Drawing for the job (mm, zero at the part's lowest x, y, z). A direction names the side the tool comes from. Coordinates: 2 decimals unless noted, no trailing zeros. Write each loop counter-clockwise with the first axis right and the second up, starting at its lowest first coordinate (ties: lowest second). Pieces come first, ordered by that corner, then holes. Notation, with made-up numbers: M 41,84 L 98,84 A24 ccw 98,104 Z; hole C 11.25,-19 d3. An arc over 180 degrees is marked long. Put each result on its own line as item: value. Start each with the question number.
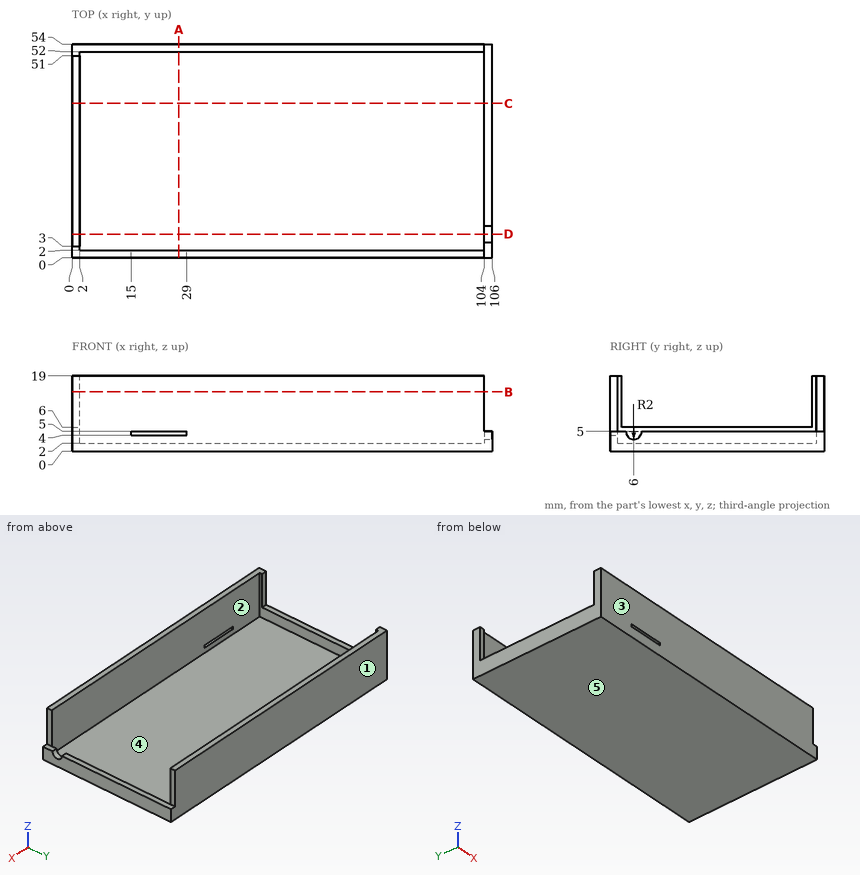
(1) Slice it at D-D, the plane y = 6. Write the cut outline in (x, z).
(2) Slice it at A-A, the plane x = 27. Write the cut outline in (y, z), then the cut area to 3 significant figures.
(3) Two-plate mould, pull along Y, no slides. Class the marked faces 1, 2 and 3: +Y half, -Y half, draft (parallel to the pull), parting line (faces both ways), or undercut.
(4) Which spindle directions (+Z, -Z, +X, -X, +Y, -Y) get a long thin tool onto all of the face, cutting with end or side? Do the marked faces 4 and 5. Say none if no direction does.
(5) Drop flat-ended pins along their axis: pin 1 (1.6 mm diameter, centred on x = 1.5, z = 15.5, fed in from -Y); pin 2 (1 mm diameter, centred on x = 66.5, y = 33.5, fed in from +Z); pin 3 (1.6 mm diameter, centred on x = 105.5, y = 41, fed in from +Z); pin 4 (2 mm diameter, centred on y = 53, z = 11.5, fed in from +X). Give the stop position or say it passes through.
(6) Slice it at C-C, the plane y = 39. Write the cut outline in (x, z), then the cut area to 3 significant figures.
(7) Drill centre lines: line 1 (Y direction, x = 88, z = 4); line 2 (Z direction, x = 99, y = 36). Where is each one in solid material? Low to high. Write a range as [from, to].
(8) Slice it at B-B, the plane z = 15. Write the cut outline in (x, y), then the cut area to 3 significant figures.
Result set:
1. outline: M 0,0 L 106,0 L 106,3 L 104,3 L 104,2 L 2,2 L 2,6 L 0,6 Z
2. outline: M 0,0 L 54,0 L 54,19 L 52,19 L 52,2 L 2,2 L 2,4 L 0,4 Z; M 0,5 L 2,5 L 2,19 L 0,19 Z
2. area: 174 mm^2
3. face 1: +Y half
3. face 2: undercut
3. face 3: -Y half
4. face 4: +Z
4. face 5: -Z, +X, -X, +Y, -Y
5. pin 1: stops at y = 0
5. pin 2: stops at z = 2
5. pin 3: stops at z = 5
5. pin 4: stops at x = 104
6. outline: M 0,0 L 106,0 L 106,5 L 104,5 L 104,2 L 2,2 L 2,6 L 0,6 Z
6. area: 226 mm^2
7. line 1: y = [0, 2], [52, 54]
7. line 2: z = [0, 2]
8. outline: M 0,0 L 104,0 L 104,2 L 2,2 L 2,3 L 0,3 Z; M 0,51 L 2,51 L 2,52 L 104,52 L 104,54 L 0,54 Z
8. area: 420 mm^2
